from build123d import *

# Parameters (mm, degrees)
SKETCH124_W             = 14.5
SKETCH124_H             = 8
PAD065_DEPTH            = 3
SKETCH125_W             = 21
SKETCH125_H             = 10
PAD066_DEPTH            = 1
SKETCH126_W             = 2
SKETCH126_H             = 5
PAD067_DEPTH            = 10
BODY024_PLACEMENT_ANGLE = 180


with BuildPart() as part:
    # Sketch124 → Pad065 (new body)
    with BuildSketch(Plane.XY):
        Rectangle(SKETCH124_W, SKETCH124_H)
    extrude(amount=PAD065_DEPTH)

    # Sketch125 → Pad066 (join)
    with BuildSketch(Plane.XY):
        with Locations((0, -1)):
            Rectangle(SKETCH125_W, SKETCH125_H)
    extrude(amount=-PAD066_DEPTH)

    # Sketch126 → Pad067 (join)
    with BuildSketch(Plane(origin=(0, 0, -1), x_dir=(1, 0, 0), z_dir=(0, 0, -1))):
        with Locations((-5.5, -1.5)):
            Rectangle(SKETCH126_W, SKETCH126_H)
        with Locations((5.5, -1.5)):
            Rectangle(SKETCH126_W, SKETCH126_H)
    extrude(amount=PAD067_DEPTH)


with BuildPart() as part_1:
    # Body024 placement: moved
    add(part.part.moved(Location((3, -13, -19.7))).rotate(Axis((3, -13, -19.7), (1, 0, 0)), BODY024_PLACEMENT_ANGLE))


solid = part_1.part
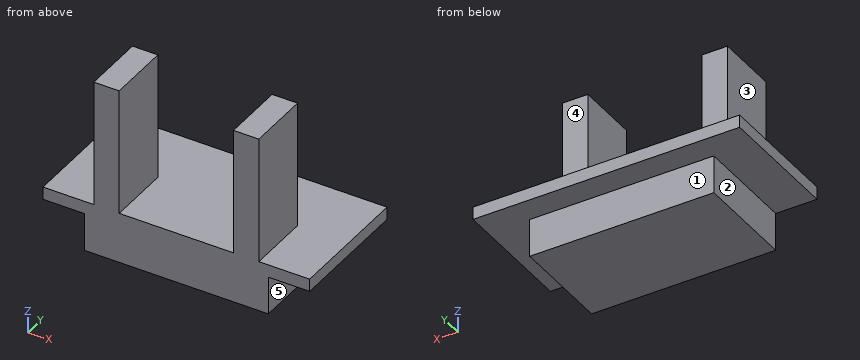
CAD build for the part. Positions are in the model's coordinates, mm. Face numbers are marked on the shaded views. A direction names the side the tool comes from. Give positions to 0.01 mm unless a question says otherwise; leave off trailing zeros. Loops run counter-clockwise (first coordinate to the right, second up) from the corner with the lowest first, then second, coordinate; pieces in that order, holes last. Notation, with made-up numbers: M 58.25,41.5 L 108.25,41.5 A31 ccw 108.25,76.5 Z; hole C 32.25,31.25 d9. An arc over 180 degrees is marked long. One line per question, with ' | ' between items. Start each with the question number.
1. 3-axis set-ups, long thin cutter, end or side, ignore diameter. For the marked faces 1, 2, 3, 4 and 5: which of +Z, -Z, +X, -X, +Y, -Y reach the whole face in a straight line?
2. Saw through at C-C on x = 0. Give the cut face in (y, z).
3. Saw through at A-A on z = -17.5. Give the cut face in (x, y).
4. Saw through at B-B on y = -13.5. Give the cut face in (x, z), plus the area to 4 significant figures.
5. Flat gauge pins, fed straight in: pin 1 (1.5 mm diameter, centred on x = 2, z = -21.5, fed in from +Y); pin 2 (4 mm diameter, centred on y = -15.5, z = -14.5, fed in from -X); pin 3 (0.9 mm diameter, centred on y = -12.5, z = -21, fed in from +X). Where does each tip first touch, or does it go through?
6. Probe L1, parallel to X at y = -15.75, z = -10; L2, parallel to Z at x = 12, y = -16.25; L3, parallel to Z at x = 0.25, y = -15.25. List the from-to ranges inside material, lowest first. Write a range as from..to.
7. Saw through at D-D on x = -3.25. Give the cut face in (y, z).
Result sheet:
1) face 1: -Z, +X, -X, +Y | face 2: -Z, -X, +Y, -Y | face 3: +Z, -X, +Y, -Y | face 4: +Z, +X, -X, +Y | face 5: -Z, +X, +Y, -Y
2) outline: M -17,-22.7 L -9,-22.7 L -9,-19.7 L -7,-19.7 L -7,-18.7 L -17,-18.7 Z
3) outline: M -3.5,-17 L -1.5,-17 L -1.5,-12 L -3.5,-12 Z; M 7.5,-17 L 9.5,-17 L 9.5,-12 L 7.5,-12 Z
4) outline: M -7.5,-19.7 L -4.25,-19.7 L -4.25,-22.7 L 10.25,-22.7 L 10.25,-19.7 L 13.5,-19.7 L 13.5,-18.7 L 9.5,-18.7 L 9.5,-8.7 L 7.5,-8.7 L 7.5,-18.7 L -1.5,-18.7 L -1.5,-8.7 L -3.5,-8.7 L -3.5,-18.7 L -7.5,-18.7 Z | area: 104.5 mm^2
5) pin 1: stops at y = -9 | pin 2: stops at x = -3.5 | pin 3: stops at x = 10.25
6) L1: x = -3.5..-1.5, 7.5..9.5 | L2: z = -19.7..-18.7 | L3: z = -22.7..-18.7
7) outline: M -17,-22.7 L -9,-22.7 L -9,-19.7 L -7,-19.7 L -7,-18.7 L -12,-18.7 L -12,-8.7 L -17,-8.7 Z
